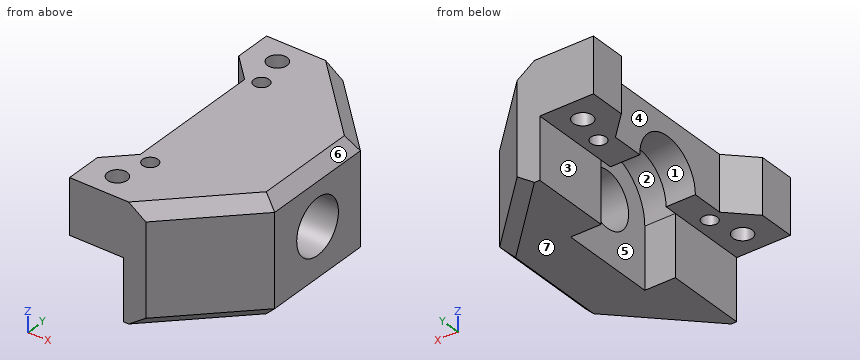
from build123d import *

# Parameters (mm, degrees)
ESQUISSE1_R                               = 1.6
BOSS_EXTRU_1_DEPTH                        = 9
ESQUISSE2_W                               = 15.7
ESQUISSE2_H                               = 42.5
BOSS_EXTRU_2_DEPTH                        = 19
ESQUISSE4_R                               = 6
ENL_V_MAT_EXTRU_1_DEPTH                   = 4.8
ENL_V_MAT_EXTRU_2_DEPTH                   = 5
ESQUISSE6_R                               = 4.5
ENL_V_MAT_EXTRU_3_DEPTH                   = 11.7
CHANFREIN1_SIZE                           = 12
CHANFREIN2_SIZE                           = 2
TROU_POUR_TARAUDAGE_POUR_TROU_TARAUD_M3_D = 2.5


with BuildPart() as part:
    # Esquisse1 → Boss.-Extru.1 (new body)
    with BuildSketch(Plane.XY):
        Polygon((38.615489841, 27.25), (38.615489841, 15.25), (38.615489841, 0), (29.815489841, 0), (29.815489841, 6), (33.815489841, 10), (33.815489841, 15.25), (33.815489841, 27.25), (33.815489841, 32.5), (29.815489841, 36.5), (29.815489841, 42.5), (38.615489841, 42.5), align=None)
        with Locations((34.615489841, 4)):
            Circle(ESQUISSE1_R, mode=Mode.SUBTRACT)
        with Locations((34.615489841, 38.5)):
            Circle(ESQUISSE1_R, mode=Mode.SUBTRACT)
    extrude(amount=BOSS_EXTRU_1_DEPTH)

    # Esquisse2 → Boss.-Extru.2 (add)
    with BuildSketch(Plane.XY.offset(9)):
        with Locations((46.465489841, 21.25)):
            Rectangle(ESQUISSE2_W, ESQUISSE2_H)
    extrude(amount=-BOSS_EXTRU_2_DEPTH)

    # Esquisse4 → Enlèv. mat.-Extru.1 (cut)
    with BuildSketch(Plane.ZY.offset(-33.815489841)):
        with Locations((0, 21.25)):
            Circle(ESQUISSE4_R)
    extrude(amount=-ENL_V_MAT_EXTRU_1_DEPTH, mode=Mode.SUBTRACT)

    # Esquisse5 → Enlèv. mat.-Extru.2 (cut)
    with BuildSketch(Plane.ZY.offset(-38.615489841)):
        with BuildLine():
            Line((0, 29.25), (-10, 29.25))
            Line((-10, 29.25), (-10, 13.25))
            Line((-10, 13.25), (0, 13.25))
            ThreePointArc((0, 13.25), (8, 21.25), (0, 29.25))
        make_face()
    extrude(amount=-ENL_V_MAT_EXTRU_2_DEPTH, mode=Mode.SUBTRACT)

    # Esquisse6 → Enlèv. mat.-Extru.3 (cut, through all)
    with BuildSketch(Plane.ZY.offset(-43.615489841)):
        with Locations((0, 21.25)):
            Circle(ESQUISSE6_R)
    extrude(amount=-ENL_V_MAT_EXTRU_3_DEPTH, mode=Mode.SUBTRACT)

    # Chanfrein1
    chanfrein1_edges = [part.edges().sort_by_distance(p)[0] for p in [
        (54.315489841, 0, -0.5),
        (54.315489841, 42.5, -0.5),
    ]]
    chamfer(chanfrein1_edges, length=CHANFREIN1_SIZE)

    # Chanfrein2
    chanfrein2_edges = [part.edges().sort_by_distance(p)[0] for p in [
        (54.315489841, 21.25, -10),
        (54.315489841, 21.25, 9),
        (48.315489841, 6, 9),
        (48.315489841, 36.5, 9),
        (48.315489841, 6, -10),
        (48.315489841, 36.5, -10),
    ]]
    chamfer(chanfrein2_edges, length=CHANFREIN2_SIZE)

    # Trou pour taraudage pour trou taraudé M31 (through all)
    with Locations(Plane.XY.offset(9)):
        with Locations((36.015489841, 33.25), (36.015489841, 9.25)):
            Hole(TROU_POUR_TARAUDAGE_POUR_TROU_TARAUD_M3_D / 2)


solid = part.part
The model under review builds one solid part; all positions refer to its coordinate system, in mm. Face numbers are marked on the shaded views. A direction names the side the tool comes from. Give positions to 0.01 mm unless a question says otherwise; leave off trailing zeros. Order: outer loops, then holes, each group sorted by start corner. A loop starts at its lowest first (then second) coordinate and runs counter-clockwise, first axis right, second up. Notation, with made-up numbers: M 37.5,74.25 L 61.5,74.25 A20 ccw 61.5,100.25 Z; hole C -27,-16.75 d9. An arc over 180 degrees is marked long. One line per question, with ' | ' between items. Start each with the question number.
1) Consider section D-D, the plane x = 51.5. Give the boundary of the cut face in (y, z), then the cut area to 3 significant figures.
2) Clearance check with flat-ended pins moving along their axes: P1, Ø1.5, axis at y = 33, z = -5.5, coming from the +X side; P2, Ø10, axis at x = 48.5, z = -1, coming from the +Y side; P3, Ø2.5, axis at x = 36, y = 34.5, coming from the -Z side; P4, Ø3, axis at x = 36.02, y = 9.25, coming from the +Z side. State where each tip first meets the part, or that it passes through.
3) Wall thickness on L1, parallel to Y at x = 34.5, z = 7; L2, parallel to Y at x = 39.75, z = -3.25; L3, parallel to Y at x = 37, z = 4.25: over which ranges is each line inside the solid? List them lowest first. Write a range as from..to.
4) Consider section A-A, the plane y = 21.25. Give the boundary of the cut face in (x, z).
5) Mouldability with a two-part tool opening along X and no side actions: class the marked faces 5, 6 and 7 as pulls with the +X half, pulls with the -X half, needs draft (parallel to the pull), parting line crosses it, or undercut.
6) For the marked faces 1, 2, 3 and 4, list the 3-axis set-ups (+Z, -Z, +X, -X, +Y, -Y) from which the entire face can be reached by the end or side of a thin tool; tool diameter is ignored.
7) Consider section B-B, the plane z = -6.25. Give the boundary of the cut face in (x, y).
8) Consider section C-C, the plane x = 34.25. Give the boundary of the cut face in (y, z).
Found:
1) outline: M 9.18,-8 L 12.01,-10 L 30.49,-10 L 33.32,-8 L 33.32,7 L 30.49,9 L 12.01,9 L 9.18,7 Z; hole C 21.25,0 d9 | area: 384 mm²
2) P1: stops at x = 52.57 | P2: stops at y = 41.32 | P3: stops at z = 0 | P4: stops at z = 9
3) L1: y = 0..2.4, 5.6..36.9, 40.1..42.5 | L2: y = 0..13.25, 29.25..42.5 | L3: y = 0..8.48, 10.02..17.01, 25.49..32.48, 34.02..42.5
4) outline: M 33.82,6 L 38.62,6 L 38.62,8 L 43.62,8 L 43.62,4.5 L 54.32,4.5 L 54.32,7 L 52.32,9 L 33.82,9 Z; M 43.62,-10 L 52.32,-10 L 54.32,-8 L 54.32,-4.5 L 43.62,-4.5 Z
5) face 5: undercut | face 6: pulls with the +X half | face 7: needs draft
6) face 1: -Z, -X | face 2: -Z | face 3: -Z, -X, +Y, -Y | face 4: +Z, -Z, -X
7) outline: M 38.62,0 L 42.32,0 L 54.32,12 L 54.32,30.5 L 42.32,42.5 L 38.62,42.5 L 38.62,29.25 L 43.62,29.25 L 43.62,13.25 L 38.62,13.25 Z
8) outline: M 0,0 L 2.44,0 L 2.44,9 L 0,9 Z; M 5.56,0 L 15.25,0 A6 cw 27.25,0 L 36.94,0 L 36.94,9 L 5.56,9 Z; M 40.06,0 L 42.5,0 L 42.5,9 L 40.06,9 Z
